from build123d import *

# Parameters (mm, degrees)
ESBO_O1_W                = 11.5
ESBO_O1_H                = 120
RESSALTO_EXTRUS_O1_DEPTH = 22.5
ESBO_O5_W                = 8.25
ESBO_O5_H                = 45
RESSALTO_EXTRUS_O2_DEPTH = 6
ESBO_O7_R                = 1.8
CORTE_EXTRUS_O1_DEPTH    = 30
CORTE_EXTRUS_O3_REACH    = 76.645
ESBO_O10_R               = 2.5
FILLET1_R                = 0.75


with BuildPart() as part:
    # Esboço1 → Ressalto-extrusão1 (new body)
    with BuildSketch(Plane(origin=(0, 0, 0), x_dir=(0, 0, -1), z_dir=(1, 0, 0))):
        with Locations((5.75, 8.378378378)):
            Rectangle(ESBO_O1_W, ESBO_O1_H)
    extrude(amount=RESSALTO_EXTRUS_O1_DEPTH)

    # Esboço5 → Ressalto-extrusão2 (add)
    with BuildSketch(Plane.ZY.offset(-8.25)):
        with Locations((4.125, -25.871621622)):
            Rectangle(ESBO_O5_W, ESBO_O5_H)
    extrude(amount=-RESSALTO_EXTRUS_O2_DEPTH)

    # Esboço7 → Corte-extrusão1 (cut)
    with BuildSketch(Plane(origin=(22.5, 0, 0), x_dir=(0, 0, -1), z_dir=(1, 0, 0))):
        with Locations((5.625, 46.878378378)):
            Circle(ESBO_O7_R)
        with Locations(Location((-4.25, -33.871621622, 0), (0, 0, 180))):
            Circle(ESBO_O7_R)
        with Locations(Location((-4.25, -25.121621622, 0), (0, 0, 180))):
            Circle(ESBO_O7_R)
        with Locations(Location((-4.25, -16.371621622, 0), (0, 0, 180))):
            Circle(ESBO_O7_R)
    extrude(amount=-CORTE_EXTRUS_O1_DEPTH, mode=Mode.SUBTRACT)

    # Corte-extrusão3: up to this face of the body (flat: up to its plane)
    corte_extrus_o3_end = Plane(part.part.faces().sort_by_distance((11.25, -25.871621622, 8.25))[0])
    # Esboço10 → Corte-extrusão3 (cut, up to the picked face)
    with BuildSketch(Plane(origin=(0, 0, -11.5), x_dir=(-1, 0, 0), z_dir=(0, 0, -1)), mode=Mode.PRIVATE) as corte_extrus_o3_sk1:
        with Locations((-11.25, -20.621621622)):
            Circle(ESBO_O10_R)
    corte_extrus_o3_tool1 = split(extrude(corte_extrus_o3_sk1.sketch, amount=-CORTE_EXTRUS_O3_REACH, mode=Mode.PRIVATE), bisect_by=corte_extrus_o3_end, keep=Keep.BOTH, mode=Mode.PRIVATE)
    add(corte_extrus_o3_tool1.solids().sort_by(Axis((11.25, -20.621622, -11.5), (0, 0, 1)))[0], mode=Mode.SUBTRACT)

    # Fillet1
    fillet1_edges = [part.edges().sort_by_distance(p)[0] for p in [
        (22.5, 68.378378378, -5.75),
        (0, 68.378378378, -5.75),
        (11.25, 68.378378378, -11.5),
        (11.25, 68.378378378, 0),
    ]]
    fillet(fillet1_edges, radius=FILLET1_R)


solid = part.part
CAD build for the part. Positions are in the model's coordinates, mm. A direction names the side the tool comes from. Coordinates: 2 decimals unless noted, no trailing zeros. Loops run counter-clockwise (first coordinate to the right, second up) from the corner with the lowest first, then second, coordinate; pieces in that order, holes last. Notation, with made-up numbers: (19, -11) - (58, -11) arc R38 cw to (58, 28) - close; hole circle Ø10 at (77.25, 54.5). An arc over 180 degrees is marked (long way). Use one line per item in the form item = value. Start each with the question number.
1) Band-saw the part on D-D (x = 17). Give the cut face in (y, z) (3 decimals).
2) Band-saw the part on A-A (x = 11.25). Give the cut face in (y, z) (3 decimals), and give its area (3 significant figures).
3) Band-saw the part on C-C (y = -29.5). Give the cut face in (x, z).
4) Band-saw the part on B-B (z = -5.75). Give the cut face in (x, y), and give its area (3 significant figures).
5) Two-plate mould, pull along X, no slides. Class faces 1 (the face through (11, -51.622, -6)), 2 (the face through (11.575, -18.143, -1.763)), 3 (the face through (8.25, -26, 2)): +X half, -X half, draft (parallel to the pull), parting line (faces both ways), or undercut.
6) Flat gauge pins, fed straight in: pin 1 (2 mm diameter, centred on y = 46.88, z = -5.62, fed in from -X); pin 2 (5 mm diameter, centred on x = 10.5, z = 3.5, fed in from +Y); pin 3 (6.5 mm diameter, centred on y = -29, z = 5, fed in from -X); pin 4 (6.5 mm diameter, centred on x = 12.5, z = 3.5, fed in from -Y). Where does each tip first touch, or does it go through?
7) Tool access for faces 4 (the face through (11.408, 48.663, -5.391)), 5 (the face through (11, -48.372, 4)), 6 (the face through (11, -3.372, 4)), 7 (the face through (14.25, -26, 2)): list every direction of +Z, -Z, +X, -X, +Y, -Y with a clear straight run to the whole face (end or side of a thin tool).
8) Drill centre lines: L1, parallel to Z at x = 1.75, y = -18; L2, parallel to Y at x = 10, z = 4.25; L3, parallel to Y at x = 9, z = -9. Where is each one in solid material? Low to high. Write a range as from..to.
Check values:
q1.outline = (-51.622, -11.5) - (67.628, -11.5) arc R0.75 ccw to (68.378, -10.75) - (68.378, -0.75) arc R0.75 ccw to (67.628, 0) - (-51.622, 0) - close; hole circle Ø3.6 at (46.878, -5.625)
q2.outline = (-51.622, -11.5) - (-23.122, -11.5) - (-23.122, 8.25) - (-48.372, 8.25) - (-48.372, 0) - (-51.622, 0) - close; (-18.122, -11.5) - (67.628, -11.5) arc R0.75 ccw to (68.378, -10.75) - (68.378, -0.75) arc R0.75 ccw to (67.628, 0) - (-3.372, 0) - (-3.372, 8.25) - (-18.122, 8.25) - (-18.122, 4.671) arc R1.8 cw (long way) to (-18.122, 3.829) - close; hole circle Ø3.6 at (-33.872, 4.25); hole circle Ø3.6 at (-25.122, 4.25); hole circle Ø3.6 at (46.878, -5.625)
q2.area = 1,610 mm2
q3.outline = (0, -11.5) - (22.5, -11.5) - (22.5, 0) - (14.25, 0) - (14.25, 8.25) - (8.25, 8.25) - (8.25, 0) - (0, 0) - close
q4.outline = (0, -51.62) - (22.5, -51.62) - (22.5, 45.08) - (0, 45.08) - close; (0, 48.67) - (22.5, 48.67) - (22.5, 67.63) arc R0.75 ccw to (21.75, 68.38) - (0.75, 68.38) arc R0.75 ccw to (0, 67.63) - close; hole circle Ø5 at (11.25, -20.62)
q4.area = 2,600 mm2
q5.face_1 = draft
q5.face_2 = undercut
q5.face_3 = -X half
q6.pin_1 = through
q6.pin_2 = -3.37
q6.pin_3 = 8.25
q6.pin_4 = -48.37
q7.face_4 = +X, -X
q7.face_5 = +Z, +X, -X, -Y
q7.face_6 = +Z, +X, -X, +Y
q7.face_7 = +Z, +X, +Y, -Y
q8.L1 = -11.5..0
q8.L2 = -48.37..-35.67, -32.07..-26.92, -23.32..-22.79, -18.46..-18.17, -14.57..-3.37
q8.L3 = -51.62..-21.71, -19.53..68.38
